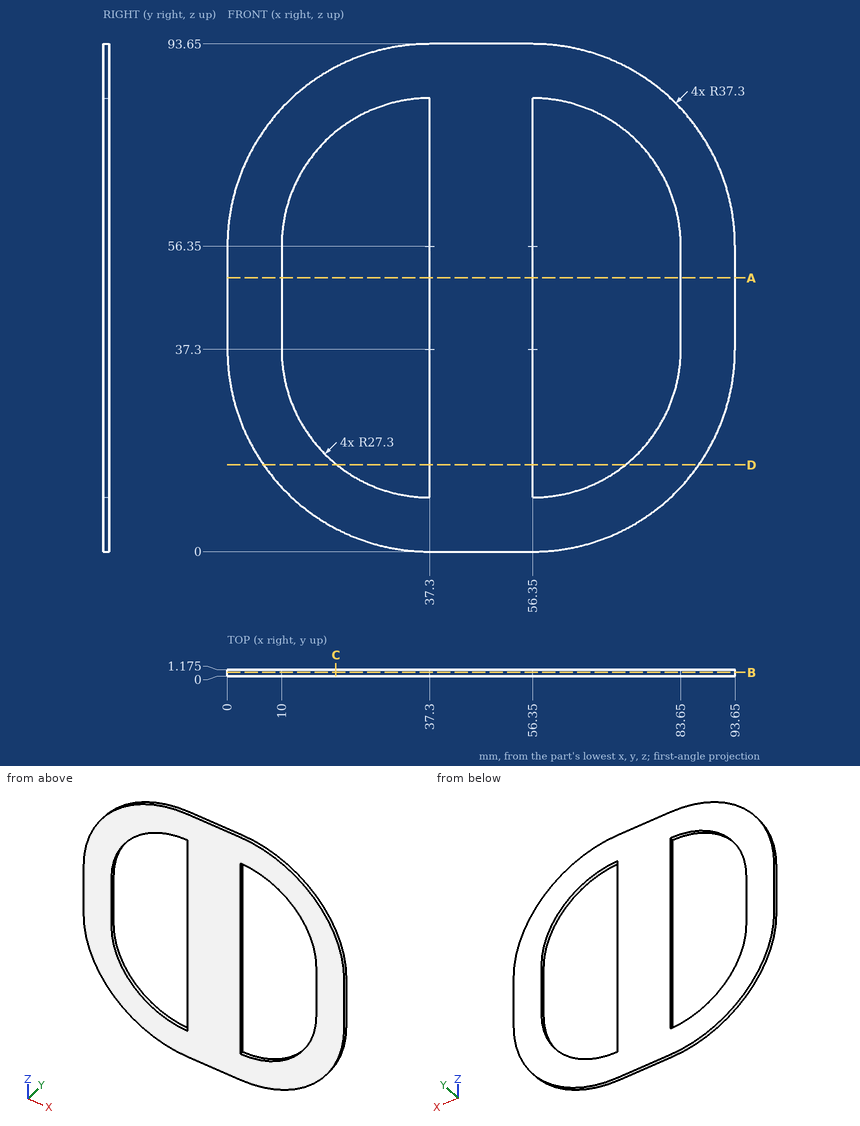
For this review, use the dimensioned drawing (mm, ordinates from the lowest corner) and the shaded views. Round coordinates to 2 decimals unless told otherwise and drop trailing zeros. Order: outer loops, then holes, each group sorted by start corner. A loop starts at its lowest first (then second) coordinate and runs counter-clockwise, first axis right, second up. Notation, with made-up numbers: (-1, 67.5) -> (54, 67.5) arc R6 cw to (54, 77.5) -> close; hole circle Ø1 at (27, 51.5). An arc over 180 degrees is marked (long way). Write item = value, one per line. Start each with the question number.
Item 1: Consider section D-D on z = 16. Write out the cut boundary in (x, y) (3 decimals).
Item 2: Consider section A-A on z = 50.5. Write out the cut boundary in (x, y) (3 decimals), plus the area to 3 significant figures.
Item 3: Consider section C-C on x = 20. Write out the cut boundary in (y, z) (3 decimals).
Item 4: Consider section B-B on y = 0.65. Write out the cut boundary in (x, z), plus the area to 3 significant figures.
Item 5: Clearance check with a flat-ended pin moving along its axis: pin 1 Ø0.6 at (y, z) = (0.5, 49) entering from -X. State where the tip first meets the part, or that it passes through.
Item 6: For line 1 along X through (y, z) = (0.3, 47); line 2 along X through (y, z) = (0.25, 32); line 3 along Z through (x, y) = (21.5, 0.2), list the stretches that pass through material, from the lowest coordinate up.
Conclusion:
q1.outline = (6.68, 0) -> (20.224, 0) -> (20.224, 1.175) -> (6.68, 1.175) -> close; (37.3, 0) -> (56.35, 0) -> (56.35, 1.175) -> (37.3, 1.175) -> close; (73.426, 0) -> (86.97, 0) -> (86.97, 1.175) -> (73.426, 1.175) -> close
q2.outline = (0, 0) -> (10, 0) -> (10, 1.175) -> (0, 1.175) -> close; (37.3, 0) -> (56.35, 0) -> (56.35, 1.175) -> (37.3, 1.175) -> close; (83.65, 0) -> (93.65, 0) -> (93.65, 1.175) -> (83.65, 1.175) -> close
q2.area = 45.9 mm2
q3.outline = (0, 4.255) -> (1.175, 4.255) -> (1.175, 16.181) -> (0, 16.181) -> close; (0, 77.469) -> (1.175, 77.469) -> (1.175, 89.395) -> (0, 89.395) -> close
q4.outline = (0, 37.3) arc R37.3 ccw to (37.3, 0) -> (56.35, 0) arc R37.3 ccw to (93.65, 37.3) -> (93.65, 56.35) arc R37.3 ccw to (56.35, 93.65) -> (37.3, 93.65) arc R37.3 ccw to (0, 56.35) -> close; hole (10, 37.3) arc R27.3 ccw to (37.3, 10) -> (37.3, 83.65) arc R27.3 ccw to (10, 56.35) -> close; hole (56.35, 10) arc R27.3 ccw to (83.65, 37.3) -> (83.65, 56.35) arc R27.3 ccw to (56.35, 83.65) -> close
q4.area = 4,190 mm2
q5.pin_1 = 0
q6.line_1 = 0 to 10, 37.3 to 56.35, 83.65 to 93.65
q6.line_2 = 0.38 to 10.52, 37.3 to 56.35, 83.13 to 93.27
q6.line_3 = 3.51 to 15.04, 78.61 to 90.14
